Could you check a few things on this model? Use its own coordinates, in mm. A direction names the side the tool comes from. Give positions to 0.01 mm unless a question says otherwise; leave off trailing zeros. Loops run counter-clockwise (first coordinate to the right, second up) from the corner with the lowest first, then second, coordinate; pieces in that order, holes last. Notation, with made-up numbers: (34.5, -12.75) - (43.5, -12.75) arc R11 ccw to (43.5, -7.75) - close; hole circle Ø8 at (56, 28.25). An arc over 180 degrees is marked (long way). One line per item, written item: value. Start each with the question number.
Q1. If I drill on line 1 (Y direction, x = 6, z = 7.5); line 2 (X direction, y = 12, z = 5); line 3 (Y direction, x = 17, z = 44.5), over which ranges is the centre line in solid material (lowest first)? Write a range as from..to.
Q2. If we mould it in two halves opening along X, with no side actions, what happens to faces 4 (the face through (3, 40.75, 6)), 5 (the face through (-6.57, 47.25, 6.34)), 6 (the face through (5, 45, 16.5))? For each: released by +X, released by -X, zero draft, split by the parting line, or undercut.
Q3. I want a section at D-D (y = -4.1). Please give me the cut outline in (x, z), then the cut area to 3 significant figures.
Q4. I want a section at C-C (z = 6). Please give me the cut outline in (x, y) (3 decimals).
Q5. I want a section at B-B (x = 4.8). Please give me the cut outline in (y, z).
Q6. I want a section at A-A (y = 34.5). Please give me the cut outline in (x, z).
Q7. I'm going to push flat-ended pins straight in: P1, Ø4, axis at x = 16, y = -4.5, coming from the +Z side; P2, Ø3, axis at x = 21, y = 17, coming from the +Z side; P3, Ø18, axis at x = 6, z = 27, coming from the +Y side. Where does each tip first touch, or does it pass through?
Q8. For faces 1 (the face through (-7.287, -11.698, 68.498)), 2 (the face through (15, 45, 16.5)), 3 (the face through (13.625, 42, 6)), which set-ups out of +Z, -Z, +X, -X, +Y, -Y let a thin tool reach every point of the face, with its end or its side?
```python
from build123d import *

# Parameters (mm, degrees)
SKETCH1_W                = 36.25
SKETCH1_H                = 56.75
SKETCH1_W_2              = 20.25
SKETCH1_H_2              = 40.75
BOSS_EXTRUDE1_DEPTH      = 12.5
SKETCH3_W                = 36.25
SKETCH3_H                = 7.5
BOSS_EXTRUDE2_DEPTH      = 56.75
BOSS_EXTRUDE2_DEPTH_BACK = 12.5
CUT_EXTRUDE1_DEPTH       = 13.5
SKETCH5_R                = 2.2
BOSS_EXTRUDE3_DEPTH      = 4
BOSS_EXTRUDE3_TAPER      = 5
FILLET1_R                = 5
FILLET2_R                = 2.5


with BuildPart() as part:
    # Sketch1 → Boss-Extrude1 (new body)
    with BuildSketch(Plane.XY):
        with Locations((10.125, 20.375)):
            Rectangle(SKETCH1_W, SKETCH1_H)
        with Locations((10.125, 20.375)):
            Rectangle(SKETCH1_W_2, SKETCH1_H_2, mode=Mode.SUBTRACT)
    extrude(amount=BOSS_EXTRUDE1_DEPTH)

    # Sketch3 → Boss-Extrude2 (add, two sides)
    with BuildSketch(Plane.XY.offset(12.5)) as boss_extrude2_sk:
        with Locations((10.125, -11.75)):
            Rectangle(SKETCH3_W, SKETCH3_H)
    extrude(amount=BOSS_EXTRUDE2_DEPTH)
    extrude(boss_extrude2_sk.sketch, amount=-BOSS_EXTRUDE2_DEPTH_BACK)

    # Sketch4 → Cut-Extrude1 (cut, through all)
    with BuildSketch(Plane.XY.offset(12.5)):
        with BuildLine():
            Line((6.625, 40.75), (13.625, 40.75))
            Line((13.625, 40.75), (13.625, 42.75))
            ThreePointArc((13.625, 42.75), (12.746320344, 44.871320344), (10.625, 45.75))
            Line((10.625, 45.75), (9.625, 45.75))
            ThreePointArc((9.625, 45.75), (7.503679656, 44.871320344), (6.625, 42.75))
            Line((6.625, 42.75), (6.625, 40.75))
        make_face()
    extrude(amount=-CUT_EXTRUDE1_DEPTH, mode=Mode.SUBTRACT)

    # Sketch5 → Boss-Extrude3 (add)
    with BuildSketch(Plane.XY.offset(12.5)):
        with Locations((4.8, 44.85)):
            Circle(SKETCH5_R)
        with Locations((15.45, 44.85)):
            Circle(SKETCH5_R)
        with Locations((15.45, -4.1)):
            Circle(SKETCH5_R)
        with Locations((4.8, -4.1)):
            Circle(SKETCH5_R)
    extrude(amount=BOSS_EXTRUDE3_DEPTH, taper=BOSS_EXTRUDE3_TAPER)

    # Fillet1
    fillet1_edges = [part.edges().sort_by_distance(p)[0] for p in [
        (-8, 48.75, 6.25),
        (28.25, 48.75, 6.25),
    ]]
    fillet(fillet1_edges, radius=FILLET1_R)

    # Fillet2
    fillet2_edges = [part.edges().sort_by_distance(p)[0] for p in [
        (-8, -11.75, 69.25),
        (28.25, -11.75, 69.25),
    ]]
    fillet(fillet2_edges, radius=FILLET2_R)


solid = part.part
```
Worked answers:
1. line 1: y = -15.5..0, 40.75..48.75
1. line 2: x = -8..0, 20.25..28.25
1. line 3: y = -15.5..-8
2. face 4: undercut
2. face 5: released by -X
2. face 6: zero draft
3. outline: (-8, 0) - (28.25, 0) - (28.25, 12.5) - (17.65, 12.5) - (17.3, 16.5) - (13.6, 16.5) - (13.25, 12.5) - (7, 12.5) - (6.65, 16.5) - (2.95, 16.5) - (2.6, 12.5) - (-8, 12.5) - close
3. area: 486 mm²
4. outline: (-8, -15.5) - (28.25, -15.5) - (28.25, 43.75) arc R5 ccw to (23.25, 48.75) - (-3, 48.75) arc R5 ccw to (-8, 43.75) - close; hole (0, 0) - (20.25, 0) - (20.25, 40.75) - (13.625, 40.75) - (13.625, 42.75) arc R3 ccw to (10.625, 45.75) - (9.625, 45.75) arc R3 ccw to (6.625, 42.75) - (6.625, 40.75) - (0, 40.75) - close
5. outline: (-15.5, 0) - (0, 0) - (0, 12.5) - (-1.9, 12.5) - (-2.25, 16.5) - (-5.95, 16.5) - (-6.3, 12.5) - (-8, 12.5) - (-8, 69.25) - (-15.5, 69.25) - close; (40.75, 0) - (48.75, 0) - (48.75, 12.5) - (47.05, 12.5) - (46.7, 16.5) - (43, 16.5) - (42.65, 12.5) - (40.75, 12.5) - close
6. outline: (-8, 0) - (0, 0) - (0, 12.5) - (-8, 12.5) - close; (20.25, 0) - (28.25, 0) - (28.25, 12.5) - (20.25, 12.5) - close
7. P1: stops at z = 16.5
7. P2: stops at z = 12.5
7. P3: stops at y = -8
8. face 1: +Z, -X, +Y, -Y
8. face 2: +Z, +X, -X, +Y
8. face 3: +Z, -Z
